```python
from build123d import *

# Parameters (mm, degrees)
ESQUISSE1_R        = 1.6
BOSS_EXTRU_1_DEPTH = 2
ESQUISSE2_R        = 0.25
BOSS_EXTRU_2_DEPTH = 5.5
ESQUISSE3_W        = 1
ESQUISSE3_H        = 3
BOSS_EXTRU_3_DEPTH = 3


with BuildPart() as part:
    # Esquisse1 → Boss.-Extru.1 (new body)
    with BuildSketch(Plane.XY):
        Polygon((0, 0), (28.7, 0), (28.7, -10), (31.7, -10), (34.7, -7.482701106), (34.7, -2.140638796), (30, 6), (0, 6), (0, 4), (4, 4), (4, 2), (0, 2), align=None)
        with Locations((31.3, -6)):
            Circle(ESQUISSE1_R, mode=Mode.SUBTRACT)
    extrude(amount=BOSS_EXTRU_1_DEPTH)

    # Esquisse2 → Boss.-Extru.2 (add)
    with BuildSketch(Plane(origin=(0, 0, 0), x_dir=(-1, 0, 0), z_dir=(0, 0, -1))):
        with Locations(Location((-28.1, 1.3, 0), (0, 0, 180))):
            Circle(ESQUISSE2_R)
        with Locations(Location((-28.1, 2.8, 0), (0, 0, 180))):
            Circle(ESQUISSE2_R)
        with Locations(Location((-26.067622213, 1.3, 0), (0, 0, 180))):
            Circle(ESQUISSE2_R)
        with Locations(Location((-26.067622213, 2.8, 0), (0, 0, 180))):
            Circle(ESQUISSE2_R)
    extrude(amount=BOSS_EXTRU_2_DEPTH)

    # Esquisse3 → Boss.-Extru.3 (add)
    with BuildSketch(Plane(origin=(0, 0, -5.5), x_dir=(-1, 0, 0), z_dir=(0, 0, -1))):
        with Locations((-28.1, 2.05)):
            Rectangle(ESQUISSE3_W, ESQUISSE3_H)
        with Locations((-26.067622213, 2.05)):
            Rectangle(ESQUISSE3_W, ESQUISSE3_H)
    extrude(amount=BOSS_EXTRU_3_DEPTH)


solid = part.part
```
Part model, mm, in its own coordinate system. A direction names the side the tool comes from. Coordinates: 2 decimals unless noted, no trailing zeros. Order: outer loops, then holes, each group sorted by start corner. A loop starts at its lowest first (then second) coordinate and runs counter-clockwise, first axis right, second up. Notation, with made-up numbers: (-19, 15) -> (1, 15) arc R19 ccw to (1, 44) -> close; hole circle Ø3 at (70, 18). An arc over 180 degrees is marked (long way). Put each result on its own line as item: value. Start each with the question number.
(1) Band-saw the part on B-B (x = 3). Give the cut face in (y, z).
(2) Band-saw the part on A-A (y = -6). Give the cut face in (x, z).
(3) Band-saw the part on D-D (x = 14). Give the cut face in (y, z).
(4) Probe line 1 along Z through (x, y) = (24, 4.25); line 2 along X through (y, z) = (3, -4.25); line 3 along Y through (x, z) = (31.3, 1.1). List the from-to ranges inside material, lowest first. Write a range as [from, to].
(5) Mould opens along X. For faces 1 (the face through (2, 2, 1)), 2 (the face through (27.6, 2, -7)), 3 (the face through (34.7, -5, 1)) say: pulls with the +X half, pulls with the -X half, needs draft (parallel to the pull), parting line crosses it, or undercut.
(6) Which spindle directions (+Z, -Z, +X, -X, +Y, -Y) get a long thin tool onto all of the face, cutting with end or side? Do faces 4 (the face through (28, 0.55, -7)), 5 (the face through (26, 3.55, -7)), 6 (the face through (28.7, -5, 1)), 7 (the face through (2, 4, 1)). Say none if no direction does.
(7) Pin check, flat tips, straight feed: pin 1 Ø0.5 at (x, z) = (28, -6.5) entering from +Y; pin 2 Ø2.5 at (y, z) = (1.5, -7) entering from +X; pin 3 Ø1.6 at (x, z) = (12.5, 1) entering from -Y. Stop position of each tip, or through.
(8) Band-saw the part on C-C (z = -1). Give the cut face in (x, y).
Determined:
1. outline: (0, 0) -> (2, 0) -> (2, 2) -> (0, 2) -> close; (4, 0) -> (6, 0) -> (6, 2) -> (4, 2) -> close
2. outline: (28.7, 0) -> (29.7, 0) -> (29.7, 2) -> (28.7, 2) -> close; (32.9, 0) -> (34.7, 0) -> (34.7, 2) -> (32.9, 2) -> close
3. outline: (0, 0) -> (6, 0) -> (6, 2) -> (0, 2) -> close
4. line 1: z = [0, 2]
4. line 2: x = [25.92, 26.22], [27.95, 28.25]
4. line 3: y = [-10, -7.6], [-4.4, 3.75]
5. face 1: needs draft
5. face 2: undercut
5. face 3: pulls with the +X half
6. face 4: -Z, +X, -X, -Y
6. face 5: -Z, +X, -X, +Y
6. face 6: +Z, -Z, -X, -Y
6. face 7: +Z, -Z, -X
7. pin 1: stops at y = 3.55
7. pin 2: stops at x = 28.6
7. pin 3: stops at y = 0
8. outline: circle Ø0.5 at (26.07, 1.3); circle Ø0.5 at (26.07, 2.8); circle Ø0.5 at (28.1, 1.3); circle Ø0.5 at (28.1, 2.8)
